Autodesk Inventor part; units mm, degrees
ref_plane "YZ Plane" through (0, 0, 0) normal (1, 0, 0) x (0, 1, 0)
ref_plane "XZ Plane" through (0, 0, 0) normal (0, 1, 0) x (-1, 0, 0)
ref_plane "XY Plane" through (0, 0, 0) normal (0, 0, 1) x (1, 0, 0)
sketch "Skizze1" plane through (0, 0, 0) normal (0, 1, 0) x (-1, 0, 0)
  line L0 (0, 0) -> (10, 0)
  line L1 (20, -14) -> (20, -70)
  line L2 (13, -70) -> (0, -70)
  line L3 (0, -70) -> (0, 0)
  line L4 (20, -70) -> (13, -70)
  line L5 (13, -70) -> (13, -93)
  line L6 (13, -93) -> (20, -93)
  line L7 (20, -93) -> (20, -70)
  line L8 (20, 0) -> (10, 0)
  line L9 (10, 0) -> (10, -14)
  line L10 (10, -14) -> (20, -14)
  line L11 (20, -14) -> (20, 0)
  line L12 (20, -12) -> (12, -12)
  line L13 (12, -12) -> (12, 0)
  line L14 (10, 2) -> (-2, 2)
  line L15 (-2, 2) -> (-2, -72)
  line L16 (-2, -72) -> (13, -72)
  line L17 (11, -70) -> (11, -95)
  line L18 (11, -95) -> (22, -95)
  line L19 (22, -95) -> (22, -70)
  line L20 (10, 2) -> (12, 2)
  line L21 (12, 2) -> (12, 0)
  line L22 (20, -12) -> (22, -12)
  line L23 (22, -12) -> (22, -70)
  line L24 (10, 0) -> (10, 2)
  line L25 (0, 0) -> (0, 2)
  line L26 (10, -14) -> (20, -14)
  line L27 (20, -14) -> (20, -21)
  line L28 (20, -21) -> (10, -21)
  line L29 (10, -21) -> (10, -14)
  line L30 (12, -12) -> (12, -14)
  line L31 (20, -21) -> (22, -21)
  line L32 (20, -14) -> (22, -14)
  line L33 (12, 2) -> (15, 2)
  line L34 (15, 2) -> (15, -14)
  line L35 (15, -14) -> (12, -14)
  line L36 (12, -14) -> (12, 2)
  line L37 (10, -14) -> (15, -14)
  line L38 (15, -14) -> (15, -21)
  line L39 (15, -21) -> (10, -21)
  line L40 (10, -21) -> (10, -14)
  point P0 (11, -72)
  dimension "d0" = 20
  dimension "d1" = 70
  dimension "d2" = 7
  dimension "d3" = 23
  dimension "d4" = 10
  dimension "d5" = 14
  dimension "d6" = 2
  dimension "d7" = 2
  dimension "d8" = 2
  dimension "d13" = 7
extrude "Extrusion1" add sketch "Skizze1" along normal blind 12 contours L3 L2 L17 L16 L15 L14 L25 | L24 L20 L21 L8 | L8 L13 L30 L10 L9 | L21 L33 L34 L8 | L8 L34 L12 L13 | L2 L5 L16 L17 | L12 L34 L10 L30 | L16 L5 L6 L7 L1 L31 L23 L19 L18 L17 | L32 L23 L31 L1
extrude "Extrusion3" add sketch "Skizze1" against normal blind 2 contours L25 L14 L24 L0 | L0 L9 L29 L28 L1 L4 L2 L3 | L3 L2 L17 L16 L15 L14 L25 | L24 L20 L21 L8 | L8 L13 L30 L10 L9 | L21 L33 L34 L8 | L8 L34 L12 L13 | L10 L38 L28 L29 | L2 L5 L16 L17 | L12 L34 L10 L30 | L4 L7 L6 L5 | L16 L5 L6 L7 L1 L31 L23 L19 L18 L17 | L10 L1 L28 L38 | L32 L23 L31 L1
chamfer "Fase1" distance 10 angle 45 1 edges at (-11, 5, -72)
fillet "Rundung1" radius 2 2 edges at (2, 5, -72) (-11, 5, -82)
fillet "Rundung2" radius 2 1 edges at (-1, 5, -72)
fillet "Rundung3" radius 2 2 edges at (-11, 5, -95) (-22, 5, -95)
fillet "Rundung4" radius 1 4 edges at (2, 5, 2) (0, 6, 2) (-10, 6, 2) (-15, 5, 2)
sketch "Skizze4" plane through (0, 12, 0) normal (0, 1, 0) x (1, 0, 0)
  line L0 (-13, 70) -> (0, 70)
  line L1 (2, -1) -> (2, 70)
  line L2 (0, 70) -> (2, 70)
  line L3 (2, 70) -> (2, 46.2)
  line L4 (2, 46.2) -> (0, 46.2)
  line L5 (0, 46.2) -> (0, 70)
  line L6 (0, 46.2) -> (2, 46.2)
  line L7 (2, 46.2) -> (2, 31.5)
  line L8 (2, 31.5) -> (0, 31.5)
  line L9 (0, 31.5) -> (0, 46.2)
  line L10 (0, 72) -> (-0.1716, 72)
  point P0 (0, 0)
  point P1 (2, 31.5)
  dimension "d24" = 14.7
  dimension "d56" = 23.8
extrude "Extrusion4" cut sketch "Skizze4" against normal blind 5.8 contours L8 L9 L4 L1
fillet "Rundung5" radius 1 1 edges at (-22, 5, -14)
sketch "Skizze5" plane through (0, -2, 0) normal (0, -1, 0) x (1, 0, 0)
  line L0 (-10, -14) -> (-15, -14)
  line L1 (-22, -15) -> (-22, -93)
  line L2 (-15, -14) -> (-22, -14)
  line L3 (-22, -14) -> (-22, -17)
  line L4 (-22, -17) -> (-15, -17)
  line L5 (-15, -17) -> (-15, -14)
  point P0 (0, 0)
  dimension "d28" = 3
extrude "Extrusion5" cut sketch "Skizze5" against normal through all
sketch "Skizze6" plane through (-10, 12, -14) normal (0, 0, -1) x (-1, 0, 0)
  line L0 (0, -12) -> (0, 0)
  line L1 (5, -12) -> (5, 0)
  line L2 (0, -12) -> (5, -12)
  line L3 (5, -12) -> (5, 0)
  line L4 (5, 0) -> (0, 0)
  line L5 (0, 0) -> (0, -12)
  point P0 (-10, -12)
extrude "Extrusion6" add sketch "Skizze6" along normal blind 3
sketch "Skizze7" plane through (0, 12, 0) normal (0, 1, 0) x (1, 0, 0)
  line L0 (-10, -1) -> (-10, 17)
  line L1 (-10, 17) -> (-13.8, 17)
  line L2 (-13.8, 17) -> (-13.8, 12)
  line L3 (-13.8, 12) -> (-10, 12)
  line L4 (-10, 12) -> (-10, 17)
  point P0 (0, 0)
  dimension "d34" = 5
  dimension "d35" = 3.8
extrude "Extrusion7" cut sketch "Skizze7" against normal up to surface (12 mm away)
sketch "Skizze8" plane through (0, 12, 0) normal (0, 1, 0) x (1, 0, 0)
  line L0 (-13, 70) -> (0, 70)
  line L1 (-13, 93) -> (-13, 70)
  point P0 (0, 0)
  point P1 (-9, 74)
  dimension "d38" = 4
  dimension "d39" = 4
hole "Bohrung1" at (-9, 12, -74) direction (0, -1, 0) diameter 2.5 end through all
sketch "Skizze9" plane through (0, 12, 0) normal (0, 1, 0) x (1, 0, 0)
  line L0 (-10, -1) -> (-10, 12)
  line L1 (-14, -2) -> (-11, -2)
  point P0 (0, 0)
  point P1 (-12.5, 5)
  dimension "d47" = 2.5
  dimension "d48" = 7
hole "Bohrung2" at (-12.5, 12, -5) direction (0, -1, 0) diameter 2.5 end through all
sketch "Skizze10" plane through (0, 12, 0) normal (0, 1, 0) x (1, 0, 0)
  line L0 (0, 70) -> (0, 46.2)
  line L1 (0, 48.85) -> (1.5, 48.85)
  line L2 (1.5, 48.85) -> (1.5, 54.35)
  line L3 (1.5, 54.35) -> (0, 54.35)
  line L4 (0, 54.35) -> (0, 48.85)
  line L5 (-13, 70) -> (0, 70)
  point P0 (0, 0)
  point P1 (0, 54.35)
  dimension "d58" = 5.5
  dimension "d59" = 1.5
  dimension "d60" = 15.65
extrude "Extrusion8" cut sketch "Skizze10" against normal up to surface (12 mm away)
sketch "Skizze11" plane through (0, 12, 0) normal (0, 1, 0) x (1, 0, 0)
  line L0 (-20, 17) -> (-20, 93)
  line L1 (-20, 17) -> (-20.5, 17)
  line L2 (-20.5, 17) -> (-20.5, 27)
  line L3 (-20.5, 27) -> (-20, 27)
  line L4 (-20, 27) -> (-20, 17)
  point P0 (0, 0)
  dimension "d63" = 0.5
  dimension "d64" = 10
extrude "Extrusion9" cut sketch "Skizze11" against normal up to surface (12 mm away)
properties part number "Case_DIP"
Build history of the part. All positions in model axes, mm. A direction names the side the tool comes from. Round coordinates to 2 decimals unless told otherwise and drop trailing zeros. Loops run counter-clockwise (first coordinate to the right, second up) from the corner with the lowest first, then second, coordinate; pieces in that order, holes last.
Item 1: Two-plate mould, pull along Z, no slides. Class faces 6 (the face through (-20, 6, -60)), 7 (the face through (-6, 5, -77)), 8 (the face through (-9.38, 4.9, -72.81)), 9 (the face through (1, 9, -46.2)): released by +Z, released by -Z, zero draft, split by the parting line, or undercut.
Item 2: Saw through at C-C (x = -9). List the corners of the cut face in (y, z), then the cut area to 3 significant figures.
Item 3: Drill centre lines: line 1 along X through (y, z) = (5.75, -5); line 2 along X through (y, z) = (7, -84); line 3 along X through (y, z) = (0.5, -61.5). Where is each one in solid material? Low to high.
Item 4: Saw through at B-B (y = 1.5). State how many separate pieces and enclosed holes the cut face has, then the cut area to 3 significant figures.
Item 5: Saw through at D-D (z = -8.5). List the corners of the cut face in (x, y).
Item 6: Which spindle directions (+Z, -Z, +X, -X, +Y, -Y) get a long thin tool onto all of the face, cutting with end or side? Do faces 1 (the face through (-11, 5, -88)), 2 (the face through (-16, 6, -93)), 3 (the face through (-13, 12, -7)), 4 (the face through (1, 9, -31.5)), 5 (the face through (-20.5, 6, -22)). Say none if no direction does.
Item 7: Saw through at A-A (z = -74). List the corners of the cut face in (x, y).
Item 8: Pin check, flat tips, straight feed: P1, Ø6, axis at x = -8.5, y = 9, coming from the -Z side; P2, Ø8, axis at x = -8.5, y = 5.5, coming from the -Z side; P3, Ø3, axis at x = -7, y = 8, coming from the +Z side; P4, Ø2, axis at x = -9, z = -74, coming from the -Y side. Stop position of each tip, or through.
Worked answers:
1. face 6: zero draft
1. face 7: released by -Z
1. face 8: undercut
1. face 9: undercut
2. outline: (-2, -80) - (12, -80) - (12, -75.25) - (-2, -75.25) - close; (-2, -72.75) - (12, -72.75) - (12, -70) - (0, -70) - (0, 2) - (-2, 2) - close
2. area: 249 mm2
3. line 1: x = -15 to -13.75, -11.25 to -10, 0 to 2
3. line 2: x = -22 to -20, -13 to -11
3. line 3: x = -22 to -20, 0 to 2
4. separate pieces: 2
4. enclosed holes: 2
4. area: 490 mm2
5. outline: (-15, -2) - (2, -2) - (2, 12) - (0, 12) - (0, 0) - (-10, 0) - (-10, 12) - (-15, 12) - close
6. face 1: -Z, +X, +Y, -Y
6. face 2: +Y
6. face 3: +Z, -Z, +X, -X, +Y
6. face 4: +X, +Y
6. face 5: +Z, +Y
7. outline: (-22, -2) - (-10.25, -2) - (-10.25, 12) - (-13, 12) - (-13, 0) - (-20, 0) - (-20, 12) - (-22, 12) - close; (-7.75, -2) - (-3, -2) - (-3, 12) - (-7.75, 12) - close
8. P1: stops at z = -94.32
8. P2: stops at z = -94.94
8. P3: stops at z = -70
8. P4: passes through
